Autodesk Inventor part; units mm, degrees
ref_plane "YZ Plane" through (0, 0, 0) normal (1, 0, 0) x (0, 1, 0)
ref_plane "XZ Plane" through (0, 0, 0) normal (0, 1, 0) x (-1, 0, 0)
ref_plane "XY Plane" through (0, 0, 0) normal (0, 0, 1) x (1, 0, 0)
sketch "Sketch1" plane through (0, 0, 0) normal (1, 0, 0) x (0, 1, 0)
  circle A0 centre (0, 0) radius 8.45
  dimension "d0" = 16.9
extrude "Extrusion1" add sketch "Sketch1" along normal mid plane 21
sketch "Sketch2" plane through (10.5, 0, 0) normal (1, 0, 0) x (0, 0, -1)
  circle A0 centre (0, 0) radius 7.725
  circle A1 centre (0, 0) radius 9.725
  dimension "d3" = 2
  dimension "d4" = 19.45
extrude "Extrusion2" cut sketch "Sketch2" against normal blind 21.5 contours A0
sketch "Sketch3" plane through (0, 0, 0) normal (0, 0, 1) x (1, 0, 0)
  circle A0 centre (0, 0) radius 5.625
  dimension "d7" = 11.25
extrude "Extrusion3" add sketch "Sketch3" along normal mid plane 18
sketch "Sketch4" plane through (0, 0, 0) normal (0, 0, 1) x (1, 0, 0)
  circle A0 centre (0, 0) radius 4.625
  dimension "d10" = 9.25
extrude "Extrusion5" cut sketch "Sketch4" along normal mid plane 100
sketch "Sketch5" plane through (10.5, 0, 0) normal (1, 0, 0) x (0, 0, -1)
  circle A0 centre (0, 0) radius 8.675
  dimension "d15" = 17.35
extrude "Extrusion6" add sketch "Sketch5" along normal blind 2
sketch "Sketch6" plane through (12.5, 0, 0) normal (1, 0, 0) x (0, 0, -1)
  arc A0 (1.0628, -4.9847) -> (6.3756, 23.0304) centre (-2.1717, 10.14) ccw
  spline S0 degree 4 poles (1.0628, -0.783) (3.325, -0.3237) (6.6509, 1.9196) (12.5543, 12.8577) (0.0955, 21.0445) (-3.8878, 23.6903) (2.1134, 24.7257) knots 0 0 0 0 0 0.38125 0.63125 1 1 1 1 1
  line L0 (-1.8785, -1.3802) -> (4.0041, -0.1858) construction
  arc A1 (-1.2523, -0.8951) -> (3.2382, 0.0167) centre (-0.4606, 6.7196) ccw construction
  spline S1 degree 2 poles (6.3756, 23.0304) (3.3857, 25.3291) (1.0628, 24.5204) knots 0 0 0 1 1 1
  line L1 (-6.8176, 23.1848) -> (11.0445, 26.2665) construction
  arc A2 (9.1477, 24.9445) -> (-4.5875, 22.5748) centre (6.4085, -0.169) ccw construction
  line L2 (-4.3138, 2.8134) -> (4.5692, 2.8134)
  line L3 (4.5692, -6.1723) -> (-4.3138, -6.1723)
  line L4 (-4.3138, -6.1723) -> (-4.3138, 2.8134)
  line L5 (4.5692, 2.8134) -> (4.5692, 1.038)
  line L6 (4.5692, -3.7804) -> (4.5692, -6.1723)
  point P0 (0, 0)
  point P1 (-0.6365, 21.8121)
  point P2 (1.0628, -0.783)
  point P3 (3.2364, 24.6304)
  point P4 (2.1134, 24.7257)
  point P5 (2.1133, 24.7254)
  point P6 (1.0633, 24.5166)
extrude "Extrusion7" add sketch "Sketch6" along normal blind 10 and the other way blind 2
sketch "Sketch7" plane through (-10.5, 0, 0) normal (-1, 0, 0) x (0, 0, 1)
  circle A0 centre (0, 0) radius 8.45
  circle A1 centre (0, 0) radius 11.1999
  dimension "d23" = 16.9
extrude "Extrusion8" cut sketch "Sketch7" against normal blind 17.75
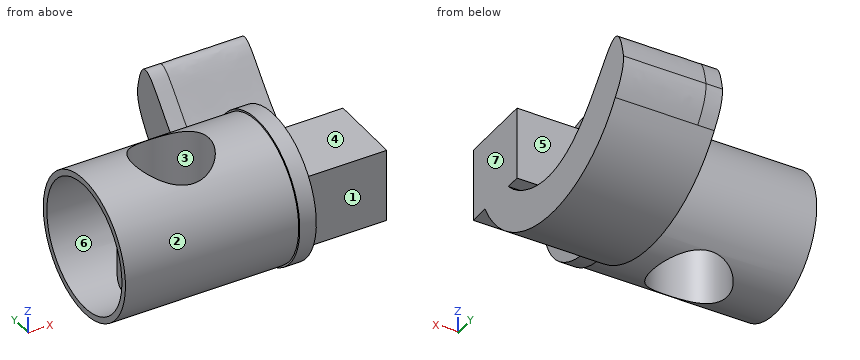
Read the model definition and answer for the solid it produces. Units are mm, in the model's axes. Face numbers are marked on the shaded views. A direction names the side the tool comes from. Give positions to 0.01 mm unless a question says otherwise; leave off trailing zeros. Order: outer loops, then holes, each group sorted by start corner. A loop starts at its lowest first (then second) coordinate and runs counter-clockwise, first axis right, second up. Notation, with made-up numbers: (-37, 81.5) -> (-1, 81.5) arc R25 cw to (-1, 93.5) -> close; hole circle Ø1 at (0, 34.5). An arc over 180 degrees is marked (long way). One line per item, written item: value. Start each with the question number.
(1) Straight lines are drawn through the part: L1, parallel to X at y = 0, z = -4 (3 decimals); L2, parallel to Y at x = 0, z = 4 (3 decimals); L3, parallel to Y at x = 1.5, z = -3.25 (3 decimals). For each, find the intervals that lie inside material, in ascending order.
(2) The part is cut by section B-B (y = 0). Determine the outline of the cut face in (x, z) (3 decimals).
(3) Flat-ended cylindrical pins translate along their axes: P1, Ø2.5, axis at x = 16, z = -0.5, coming from the +Y side; P2, Ø5, axis at x = -4.5, z = -9.5, coming from the +Y side; P3, Ø1, axis at x = 4, z = 4.5, coming from the +Y side; P4, Ø10, axis at x = 15.5, z = -1.5, coming from the -Y side (3 decimals). Find the tip coordinate at first contact, or state that the pin passes through.
(4) A tool of negligible diameter and unlimited length cuts with its end or side. For the marked faces 1, 2, 3 and 4, from which of +Z, -Z, +X, -X, +Y, -Y can it reach the whole face along a straight path? Write none if from no direction.
(5) For a pull along X with two mould halves and no side action, classify the marked faces 5, 6 and 7 as released by +X, released by -X, zero draft, split by the parting line, or undercut.
(6) The part is cut by section C-C (z = 5.25). Determine the outline of the cut face in (x, y) (3 decimals), and give its area (3 significant figures).
(7) The part is cut by section A-A (x = 0). Determine the outline of the cut face in (y, z) (3 decimals).
(8) The part is cut by section D-D (z = 0). State how many separate pieces and enclosed holes the cut face has, and give its area (3 significant figures).
Taken from the geometry:
1. L1: -5.625 to -4.625, 4.625 to 5.625, 10.5 to 22.5
1. L2: -7.443 to -6.609, -5.625 to -4.625, 4.625 to 5.625, 6.609 to 7.443
1. L3: -7.8 to -7.008, -5.421 to -4.375, 4.375 to 5.421, 7.008 to 7.8
2. outline: (-10.5, -8.45) -> (-4.625, -8.45) -> (-4.625, 8.45) -> (-10.5, 8.45) -> (-10.5, 7.725) -> (-5.625, 7.725) -> (-5.625, -7.725) -> (-10.5, -7.725) -> close; (4.625, -8.45) -> (10.5, -8.45) -> (10.5, -9.507) -> (22.5, -9.507) -> (22.5, 4.314) -> (12.5, 4.314) -> (12.5, 8.675) -> (10.5, 8.675) -> (10.5, 8.45) -> (4.625, 8.45) -> close; hole (5.625, -7.725) -> (10.5, -7.725) -> (10.5, 7.725) -> (5.625, 7.725) -> close
3. P1: y = 24.66
3. P2: y = 4.73
3. P3: y = 7.44
3. P4: y = -8.675
4. face 1: +Z, -Z, +X, -Y
4. face 2: -X
4. face 3: +Z, -Z
4. face 4: +Z, +X, +Y, -Y
5. face 5: zero draft
5. face 6: undercut
5. face 7: released by +X
6. outline: (-10.5, -6.621) -> (10.5, -6.621) -> (10.5, -6.906) -> (12.5, -6.906) -> (12.5, 6.906) -> (10.5, 6.906) -> (10.5, 6.621) -> (-10.5, 6.621) -> (-10.5, 5.667) -> (10.5, 5.667) -> (10.5, -5.667) -> (-10.5, -5.667) -> close; circle Ø11.25 at (0, 0); hole circle Ø9.25 at (0, 0)
6. area: 99.9 mm^2
7. outline: (-4.625, -7.072) -> (-4.625, 7.072) arc R8.45 ccw to start; (4.625, -7.072) arc R8.45 ccw to (4.625, 7.072) -> close; hole (-5.625, -5.295) -> (-5.625, 5.295) arc R7.725 ccw to start; hole (5.625, -5.295) arc R7.725 ccw to (5.625, 5.295) -> close
8. separate pieces: 3
8. enclosed holes: 1
8. area: 224 mm^2
